Geometry check sheet. Reference: the model listing, model coordinates, mm. Coordinates: 2 decimals unless noted, no trailing zeros. Use CSV: the item, a comma, the result in double quotes. Start each with the question number.
1) Sectioned sample at A-A, the plane x = -195. Count the separate pieces of the cut face and the enclosed holes in it, and give its area (3 significant figures).
2) Depth check by flat-ended pin: P1, Ø10, axis at x = -204.5, z = 5.5, coming from the +Y side; P2, Ø3, axis at x = -158, z = 31.5, coming from the +Y side. Enter the tip coordinate at first touch or a pass-through.
3) Thickness scan on probe 1 along Z at (x, y) = (-203.2, -13.75) (3 decimals); probe 2 along Z at (x, y) = (187.5, -17.75); probe 3 along Z at (x, y) = (-126.5, -13.5). Record the ranges inside material, lowest first. Write a range as [from, to].
from build123d import *

# Parameters (mm, degrees)
F0_W     = 614.6593689919
F0_H     = 104.9060299742
F0_R     = 20.32
F1_DEPTH = 25.4


# Not quite as in the source:
# - ends of sketch curves that miss each other by under 0.0002 mm in the source are joined
# - the dataset's text gives a spline's control points without its knots; the knots are read off the source's solid


with BuildPart() as f1:
    # F0 (on Front) → F1 (new body)
    with BuildSketch(Plane.XZ):
        with Locations((0, 30.0749056167)):
            Rectangle(F0_W, F0_H)
        with Locations((-203.2, 20.4950086772)):
            Circle(F0_R, mode=Mode.SUBTRACT)
        with Locations((0, 20.4950086772)):
            Circle(F0_R, mode=Mode.SUBTRACT)
        with Locations((203.2, 20.4950086772)):
            Circle(F0_R, mode=Mode.SUBTRACT)
        with BuildLine():
            add(Edge.make_bspline(
                [(0, 63.5), (50.8, 63.5), (56.1175370932, 0), (101.6, 0)],
                knots=[0, 0, 0, 0, 119.8115603771, 119.8115603771, 119.8115603771, 119.8115603771], degree=3))
            add(Edge.make_bspline(
                [(0, 63.5), (-50.8, 63.5), (-56.1175370932, 0), (-101.6, 0)],
                knots=[0, 0, 0, 0, 119.8115603771, 119.8115603771, 119.8115603771, 119.8115603771], degree=3))
            add(Edge.make_bspline(
                [(-101.6, 0), (-147.0824629068, 0), (-161.2765789032, 63.5), (-203.2, 63.5)],
                knots=[0, 0, 0, 0, 119.8115603771, 119.8115603771, 119.8115603771, 119.8115603771], degree=3))
            add(Edge.make_bspline(
                [(-203.2, 63.5), (-244.3384826183, 63.5), (-263.5250381589, 4.789814353), (-266.7, 0)],
                knots=[0, 0, 0, 0, 89.8025612107, 89.8025612107, 89.8025612107, 89.8025612107], degree=3))
            Line((-266.7, 0), (-270.9370674539, 2.8072381066))
            add(Edge.make_bspline(
                [(-203.2, 68.58), (-206.0749247482, 68.58), (-211.6570572562, 68.0654677515), (-219.449703116, 65.9327946823), (-226.6139167838, 62.6573237184), (-235.3214664022, 57.0619610705), (-242.8084043286, 50.0452799381), (-249.2087272272, 42.3342188514), (-253.4945356129, 36.3678079721), (-257.2899146838, 30.3831174449), (-260.614540304, 24.5429222876), (-263.4845904473, 19.0110013278), (-265.5085267197, 14.7960229142), (-266.9118861506, 11.7464153334), (-267.8572021622, 9.6427688992), (-268.6955290239, 7.7460864416), (-269.4259857327, 6.0820696315), (-269.9424600992, 4.9140477877), (-270.2959565612, 4.1311962061), (-270.5287914392, 3.627286717), (-270.6926175205, 3.2849255658), (-270.8015436387, 3.065424442), (-270.8703935577, 2.930969375), (-270.9134306119, 2.8501874319), (-270.9322031409, 2.8160102358), (-270.9370674539, 2.8072381066)],
                knots=[0, 0, 0, 0, 0.062536818, 0.125073636, 0.1876104541, 0.2501472721, 0.3752209081, 0.4377577261, 0.5002945442, 0.5628313622, 0.6253681802, 0.6879049982, 0.7504418162, 0.7817102252, 0.8129786342, 0.8442470433, 0.8755154523, 0.9067838613, 0.9224180658, 0.9380522703, 0.9536864748, 0.961503577, 0.9693206793, 0.9771377815, 0.9803545729, 0.9803545729, 0.9803545729, 0.9803545729], degree=3))
            add(Edge.make_bspline(
                [(-101.6, 5.08), (-104.1471371, 5.08), (-108.9825494519, 5.5227985642), (-115.6526939013, 7.3372474831), (-121.9092103663, 10.1773367447), (-127.8642663749, 13.932751749), (-133.5886395499, 18.4728381682), (-140.9907545945, 25.3635161712), (-149.9577750737, 35.1135642507), (-159.0396450213, 45.1591389287), (-166.7656656648, 52.6297090899), (-172.9079254728, 57.7563865096), (-179.5208319726, 62.1967681684), (-186.7206430613, 65.7097554828), (-194.5808153214, 68.0207957165), (-200.2591817799, 68.58), (-203.2, 68.58)],
                knots=[0, 0, 0, 0, 0.0625, 0.125, 0.1875, 0.25, 0.3125, 0.375, 0.5, 0.625, 0.6875, 0.75, 0.8125, 0.875, 0.9375, 1, 1, 1, 1], degree=3))
            add(Edge.make_bspline(
                [(0, 68.58), (-3.4395833333, 68.58), (-9.9907230249, 68.0415568729), (-18.8754835158, 65.7852306257), (-26.8494717203, 62.2976627153), (-33.979773011, 57.8349170952), (-40.3831564519, 52.6526314317), (-48.14551851, 45.0924908704), (-56.7790114699, 34.9489891198), (-64.9188221861, 25.1689190997), (-71.5831601125, 18.303665252), (-76.7480703911, 13.8055020439), (-82.1704530142, 10.1054105506), (-87.9633960673, 7.3142638881), (-94.302168804, 5.5228017002), (-99.0528629, 5.08), (-101.6, 5.08)],
                knots=[0, 0, 0, 0, 0.0625, 0.125, 0.1875, 0.25, 0.3125, 0.375, 0.5, 0.625, 0.6875, 0.75, 0.8125, 0.875, 0.9375, 1, 1, 1, 1], degree=3))
            add(Edge.make_bspline(
                [(0, 68.58), (3.4395833333, 68.58), (9.9907230249, 68.0415568729), (18.8754835158, 65.7852306257), (26.8494717203, 62.2976627153), (33.979773011, 57.8349170952), (40.3831564519, 52.6526314317), (48.14551851, 45.0924908704), (56.7790114699, 34.9489891198), (64.9188221861, 25.1689190997), (71.5831601125, 18.303665252), (76.7480703911, 13.8055020439), (82.1704530142, 10.1054105506), (87.9633960673, 7.3142638881), (94.302168804, 5.5228017002), (99.0528629, 5.08), (101.6, 5.08)],
                knots=[0, 0, 0, 0, 0.0625, 0.125, 0.1875, 0.25, 0.3125, 0.375, 0.5, 0.625, 0.6875, 0.75, 0.8125, 0.875, 0.9375, 1, 1, 1, 1], degree=3))
            add(Edge.make_bspline(
                [(101.6, 5.08), (104.1471371, 5.08), (108.9825494519, 5.5227985642), (115.6526939013, 7.3372474831), (121.9092103663, 10.1773367447), (127.8642663749, 13.932751749), (133.5886395499, 18.4728381682), (140.9907545945, 25.3635161712), (149.9577750737, 35.1135642507), (159.0396450213, 45.1591389287), (166.7656656648, 52.6297090899), (172.9079254728, 57.7563865096), (179.5208319726, 62.1967681684), (186.7206430613, 65.7097554828), (194.5808153214, 68.0207957165), (200.2591817799, 68.58), (203.2, 68.58)],
                knots=[0, 0, 0, 0, 0.0625, 0.125, 0.1875, 0.25, 0.3125, 0.375, 0.5, 0.625, 0.6875, 0.75, 0.8125, 0.875, 0.9375, 1, 1, 1, 1], degree=3))
            add(Edge.make_bspline(
                [(203.2, 68.58), (206.0749247482, 68.58), (211.6570572562, 68.0654677515), (219.449703116, 65.9327946823), (226.6139167838, 62.6573237184), (235.3214664022, 57.0619610705), (242.8084043286, 50.0452799381), (249.2087272272, 42.3342188514), (253.4945356129, 36.3678079721), (257.2899146838, 30.3831174449), (260.614540304, 24.5429222876), (263.4845904473, 19.0110013278), (265.5085267197, 14.7960229142), (266.9118861506, 11.7464153334), (267.8572021622, 9.6427688992), (268.6955290239, 7.7460864416), (269.4259857327, 6.0820696315), (269.9424600992, 4.9140477877), (270.2959565612, 4.1311962061), (270.5287914392, 3.627286717), (270.6926175205, 3.2849255658), (270.8015436387, 3.065424442), (270.8703935577, 2.930969375), (270.9134306119, 2.8501874319), (270.9322031409, 2.8160102358), (270.9370672724, 2.8072380059)],
                knots=[0, 0, 0, 0, 0.062536818, 0.125073636, 0.1876104541, 0.2501472721, 0.3752209081, 0.4377577261, 0.5002945442, 0.5628313622, 0.6253681802, 0.6879049982, 0.7504418162, 0.7817102252, 0.8129786342, 0.8442470433, 0.8755154523, 0.9067838613, 0.9224180658, 0.9380522703, 0.9536864748, 0.961503577, 0.9693206793, 0.9771377815, 0.9803545729, 0.9803545729, 0.9803545729, 0.9803545729], degree=3))
            Line((270.9370672724, 2.8072380059), (266.7, 0))
            add(Edge.make_bspline(
                [(203.2, 63.5), (244.3384826183, 63.5), (263.5250381589, 4.789814353), (266.7, 0)],
                knots=[0, 0, 0, 0, 89.8025612107, 89.8025612107, 89.8025612107, 89.8025612107], degree=3))
            add(Edge.make_bspline(
                [(101.6, 0), (147.0824629068, 0), (161.2765789032, 63.5), (203.2, 63.5)],
                knots=[0, 0, 0, 0, 119.8115603771, 119.8115603771, 119.8115603771, 119.8115603771], degree=3))
        make_face(mode=Mode.SUBTRACT)
    extrude(amount=F1_DEPTH)


solid = f1.part
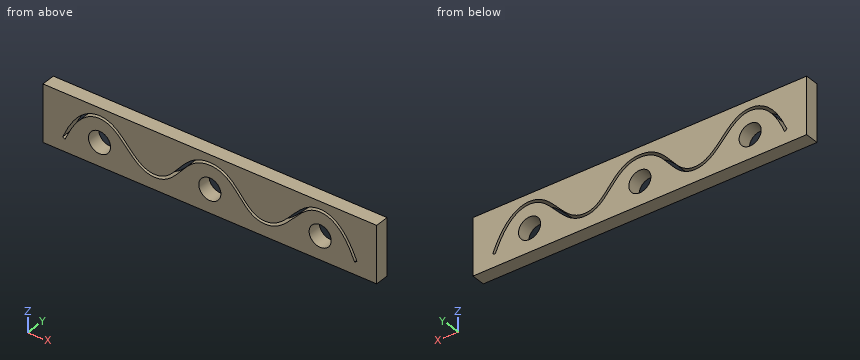
Evaluation:
1,separate pieces,"3"
1,enclosed holes,"0"
1,area,"1,590 mm²"
2,P1,"through"
2,P2,"y = 0"
3,probe 1,"[-22.378, 0.175], [40.815, 63.5], [68.58, 82.528]"
3,probe 2,"[-22.38, 7.59], [33.4, 60.3], [65.76, 82.53]"
3,probe 3,"[-22.38, 7.13], [13.15, 82.53]"
